For this review, use the dimensioned drawing (mm, ordinates from the lowest corner) and the shaded views. A direction names the side the tool comes from. Give positions to 0.01 mm unless a question says otherwise; leave off trailing zeros. Loops run counter-clockwise (first coordinate to the right, second up) from the corner with the lowest first, then second, coordinate; pieces in that order, holes last. Notation, with made-up numbers: (32.5, 30) - (75.5, 30) arc R17 ccw to (75.5, 53) - close; hole circle Ø9 at (-4.5, 44.25). An arc over 180 degrees is marked (long way). Put each result on its own line as item: value.
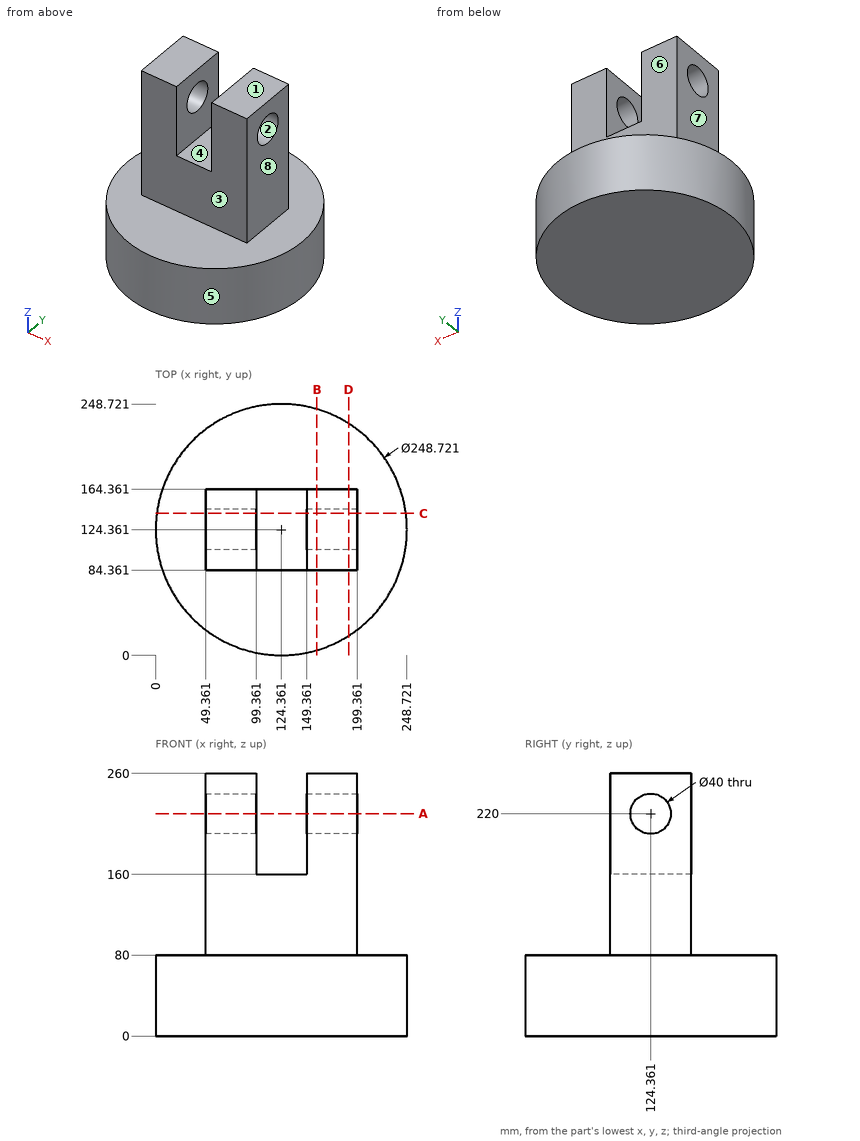
1) Take a section at D-D on x = 191. State the section outline as (y, z) points, and give its area (3 significant figures).
Geometry check:
outline: (19.36, 0) - (229.36, 0) - (229.36, 80) - (164.36, 80) - (164.36, 260) - (84.36, 260) - (84.36, 80) - (19.36, 80) - close; hole circle Ø40 at (124.36, 220)
area: 29,900 mm²
2) Take a section at A-A on z = 220. State the section outline as (x, y) points, and give its area (3 significant figures).
Geometry check:
outline: (49.36, 84.36) - (99.36, 84.36) - (99.36, 104.36) - (49.36, 104.36) - close; (49.36, 144.36) - (99.36, 144.36) - (99.36, 164.36) - (49.36, 164.36) - close; (149.36, 84.36) - (199.36, 84.36) - (199.36, 104.36) - (149.36, 104.36) - close; (149.36, 144.36) - (199.36, 144.36) - (199.36, 164.36) - (149.36, 164.36) - close
area: 4,000 mm²
3) Draft analysis for pull direction Z (two halves, no side actions). For the marked faces 1, 2 and 3, state which applies: pulls with the +Z half, pulls with the -Z half, needs draft (parallel to the pull), parting line crosses it, or undercut.
Geometry check:
face 1: pulls with the +Z half
face 2: undercut
face 3: needs draft
4) Take a section at C-C on y = 140.5. State the section outline as (x, z) points.
Geometry check:
outline: (1.05, 0) - (247.67, 0) - (247.67, 80) - (199.36, 80) - (199.36, 208.19) - (149.36, 208.19) - (149.36, 160) - (99.36, 160) - (99.36, 208.19) - (49.36, 208.19) - (49.36, 80) - (1.05, 80) - close; (49.36, 231.81) - (99.36, 231.81) - (99.36, 260) - (49.36, 260) - close; (149.36, 231.81) - (199.36, 231.81) - (199.36, 260) - (149.36, 260) - close
5) For the marked faces 4, 5, 6, 7 and 8, list the 3-axis set-ups (+Z, -Z, +X, -X, +Y, -Y) from which the entire face can be reached by the end or side of a thin tool; tool diameter is ignored.
Geometry check:
face 4: +Z, +Y, -Y
face 5: +Z, -Z
face 6: +Z, +X, -X, +Y
face 7: +Z, -X, +Y, -Y
face 8: +Z, +X, +Y, -Y
6) Wall thickness on line 1 (Y direction, x = 179.5, z = 220); line 2 (X direction, y = 147, z = 220); line 3 (X direction, y = 138.5, z = 94.5): over which ranges is each line inside the solid? List them lowest first.
Geometry check:
line 1: y = 84.36 to 104.36, 144.36 to 164.36
line 2: x = 49.36 to 99.36, 149.36 to 199.36
line 3: x = 49.36 to 199.36
7) Insertion check: pin 1 Ø24 at (y, z) = (122, 210.5) entering from -X; pin 2 Ø2 at (y, z) = (114.5, 34.5) entering from +X (1 decimal); pin 3 Ø2 at (x, y) = (211.5, 133.5) entering from +Z. Each pin has a flat end and moves straight along its axis. Give the tip position at first contact, or say it passes through.
Geometry check:
pin 1: stops at x = 49.36
pin 2: stops at x = 248.4
pin 3: stops at z = 80
8) Take a section at B-B on x = 159.5. State the section outline as (y, z) points, and give its area (3 significant figures).
Geometry check:
outline: (5.07, 0) - (243.65, 0) - (243.65, 80) - (164.36, 80) - (164.36, 260) - (84.36, 260) - (84.36, 80) - (5.07, 80) - close; hole circle Ø40 at (124.36, 220)
area: 32,200 mm²
